Part model, mm, in its own coordinate system. A direction names the side the tool comes from. Give positions to 0.01 mm unless a question says otherwise; leave off trailing zeros. Order: outer loops, then holes, each group sorted by start corner. A loop starts at its lowest first (then second) coordinate and runs counter-clockwise, first axis right, second up.
1. Slice it at D-D on z = -0.5. List the corners of the cut face in (x, y).
2. Slice it at A-A on y = -1.5. List the corners of the cut face in (x, z), and give its area (3 significant figures).
3. Which spindle directions (+Z, -Z, +X, -X, +Y, -Y) get a long thin tool onto all of the face, cutting with end or side? Do faces 1 (the flat face through (0, 1, 1.65)), 2 (the flat face through (-3.21, 3.5, 0.44)). Say none if no direction does.
4. Slice it at C-C on y = 1.75. List the corners of the cut face in (x, z).
5. Drop flat-ended pins along their axis: pin 1 Ø0.6 at (x, y) = (0, -1) entering from +Z; pin 2 Ø0.6 at (y, z) = (-1.5, 0) entering from +X; pin 3 Ø1 at (y, z) = (1, 1) entering from -X. Give the stop position or say it passes through.
6. Probe line 1 (Z direction, x = 2.5, y = -2); line 2 (Y direction, x = 0.75, z = -1.25); line 3 (Z direction, x = -2, y = 2.25). List the from-to ranges inside material, lowest first.
7. Slice it at B-B on x = 1.75. List the corners of the cut face in (y, z), and give its area (3 significant figures).
from build123d import *
from OCP.BRepFilletAPI import BRepFilletAPI_MakeChamfer

# Parameters (mm, degrees)
ESBO_O1_W                = 6.7
ESBO_O1_H                = 3.3
RESSALTO_EXTRUS_O1_DEPTH = 7.1
ESBO_O2_W                = 6.7
ESBO_O2_H                = 4.1
CORTE_EXTRUS_O1_DEPTH    = 0.7
REVOLU_O1_ANGLE          = 180
ESBO_O4_W                = 0.5
ESBO_O4_H                = 0.5
RESSALTO_EXTRUS_O2_DEPTH = 3
CHANFRO1_SIZE            = 0.3
CHANFRO1_SIZE_2          = 0.824243226
CHANFRO2_SIZE            = 2
CHANFRO2_SIZE2           = 0.352653961


with BuildPart() as part:
    # Esboço1 → Ressalto-extrusão1 (new body)
    with BuildSketch(Plane(origin=(0, 0, 0), x_dir=(1, 0, 0), z_dir=(0, 1, 0))):
        Rectangle(ESBO_O1_W, ESBO_O1_H)
    extrude(amount=RESSALTO_EXTRUS_O1_DEPTH)

    # Esboço2 → Corte-extrusão1 (cut)
    with BuildSketch(Plane.XY.offset(1.65)):
        with Locations((0, 5.05)):
            Rectangle(ESBO_O2_W, ESBO_O2_H)
    extrude(amount=-CORTE_EXTRUS_O1_DEPTH, mode=Mode.SUBTRACT)

    # Esboço3 → Revolução1 (revolve)
    with BuildSketch(Plane.XY.offset(0.95)):
        with BuildLine():
            Line((0, 6.911003495), (0, 3.188996505))
            ThreePointArc((0, 3.188996505), (1.861003495, 5.05), (0, 6.911003495))
        make_face()
    revolve(axis=Axis((0, 7.1, 0.95), (0, -1, 0)), revolution_arc=REVOLU_O1_ANGLE)

    # Esboço4 → Ressalto-extrusão2 (add)
    with BuildSketch(Plane.XZ):
        Rectangle(ESBO_O4_W, ESBO_O4_H)
        with Locations((-2.54, 0)):
            Rectangle(ESBO_O4_W, ESBO_O4_H)
        with Locations((2.54, 0)):
            Rectangle(ESBO_O4_W, ESBO_O4_H)
    extrude(amount=RESSALTO_EXTRUS_O2_DEPTH)

    # Chanfro1
    # the kernel refuses this chamfer: 0.824243226, 0.3 mm, written as the material it takes off along each edge
    with BuildSketch(Plane(origin=(5.488247435, 3, 1.65), x_dir=(0, -0.9950833631817485, 0.09904090225205103), z_dir=(-1, 0, 0))) as chanfro1_piece_1_section:
        Polygon((CHANFRO1_SIZE * 0.995083363182, -CHANFRO1_SIZE * 0.0990409022521), (-CHANFRO1_SIZE_2 * 0.0990409022324, -CHANFRO1_SIZE_2 * 0.995083362984), (0, 0), align=None)
    chanfro1_piece_1 = extrude(amount=10.97649487, mode=Mode.PRIVATE)
    chanfro1_piece_1 = split(chanfro1_piece_1, bisect_by=Plane(origin=(0, 2.90340276, 0.95), z_dir=(0, 0, 1)), keep=Keep.TOP, mode=Mode.PRIVATE)
    add(chanfro1_piece_1, mode=Mode.SUBTRACT)

    # Chanfro2: one chamfer whose edges measure the first distance from different faces: ONE call of the kernel's chamfer builder (chamfer() names one face for all edges)
    chanfro2_edges_1 = [part.edges().sort_by_distance(p)[0] for p in [
        (3.35, 1.35, 1.65),
    ]]
    chanfro2_side_1 = [part.faces().sort_by_distance(p)[0] for p in [
        (3.35, 3.34322922, -0.190735653),
    ]]
    chanfro2_edges_2 = [part.edges().sort_by_distance(p)[0] for p in [
        (-3.35, 1.35, 1.65),
    ]]
    chanfro2_side_2 = [part.faces().sort_by_distance(p)[0] for p in [
        (-3.35, 3.34322922, -0.190735653),
    ]]
    chanfro2 = BRepFilletAPI_MakeChamfer(part.part.solid().wrapped)
    for e in chanfro2_edges_1:
        chanfro2.Add(CHANFRO2_SIZE, CHANFRO2_SIZE2, e.wrapped, chanfro2_side_1[0].wrapped)  # the first distance lies on this face
    for e in chanfro2_edges_2:
        chanfro2.Add(CHANFRO2_SIZE, CHANFRO2_SIZE2, e.wrapped, chanfro2_side_2[0].wrapped)  # the first distance lies on this face
    add(Compound.cast(chanfro2.Shape()), mode=Mode.REPLACE)


solid = part.part
Data:
1. outline: (-3.35, 0) - (3.35, 0) - (3.35, 7.1) - (-3.35, 7.1) - close
2. outline: (-2.79, -0.25) - (-2.29, -0.25) - (-2.29, 0.25) - (-2.79, 0.25) - close; (-0.25, -0.25) - (0.25, -0.25) - (0.25, 0.25) - (-0.25, 0.25) - close; (2.29, -0.25) - (2.79, -0.25) - (2.79, 0.25) - (2.29, 0.25) - close
2. area: 0.750 mm2
3. face 1: +Z, +X, -X, -Y
3. face 2: +Z, -X, +Y, -Y
4. outline: (-3.35, -1.65) - (3.35, -1.65) - (3.35, -0.35) - (3, 1.65) - (-3, 1.65) - (-3.35, -0.35) - close
5. pin 1: stops at z = 0.25
5. pin 2: stops at x = 2.79
5. pin 3: stops at x = -3.2
6. line 1: z = -0.25 to 0.25
6. line 2: y = 0 to 7.1
6. line 3: z = -1.65 to 1.65
7. outline: (0, -1.65) - (7.1, -1.65) - (7.1, 0.95) - (5.68, 0.95) arc R0.63 ccw to (4.42, 0.95) - (2.95, 0.95) - (2.7, 1.65) - (0, 1.65) - close
7. area: 21.1 mm2
